Verification items for the finished model (mm, model axes). Face numbers are marked on the shaded views. A direction names the side the tool comes from. Round coordinates to 2 decimals unless told otherwise and drop trailing zeros. Loops run counter-clockwise (first coordinate to the right, second up) from the corner with the lowest first, then second, coordinate; pieces in that order, holes last. Notation, with made-up numbers: M 24,6 L 58,6 A17 cw 58,29 Z; hole C -7,65.5 d7. An arc over 180 degrees is marked long. One line per item, written item: value.
from build123d import *

# Parameters (mm, degrees)
F0_R      = 1.6
F1_DEPTH  = 1.6
F2_W      = 5.5
F2_H      = 10.75
F2_W_2    = 6.8
F2_H_2    = 5.8
F3_DEPTH  = 3.6
F2_W_3    = 8.75
F2_H_3    = 16.2
F4_DEPTH  = 9
F5_DEPTH  = 2
F7_DEPTH  = 2
F6_W      = 8.5
F6_H      = 0.6
F6_H_2    = 9
F8_DEPTH  = 4.25
F6_W_2    = 5.3
F6_H_3    = 6.7
F9_DEPTH  = 3.4
F6_W_3    = 8
F6_H_4    = 7
F10_DEPTH = 4


with BuildPart() as f1:
    # F0 (on Top) → F1 (new body)
    with BuildSketch(Plane.XY):
        with BuildLine():
            Line((15.6, 18.1), (-15.6, 18.1))
            ThreePointArc((-15.6, 18.1), (-17.367767, 17.367767), (-18.1, 15.6))
            Line((-18.1, 15.6), (-18.1, -15.6))
            ThreePointArc((-18.1, -15.6), (-17.367767, -17.367767), (-15.6, -18.1))
            Line((-15.6, -18.1), (15.6, -18.1))
            ThreePointArc((15.6, -18.1), (17.367767, -17.367767), (18.1, -15.6))
            Line((18.1, -15.6), (18.1, 15.6))
            ThreePointArc((18.1, 15.6), (17.367767, 17.367767), (15.6, 18.1))
        make_face()
        with Locations((-15.6, -15.6)):
            Circle(F0_R, mode=Mode.SUBTRACT)
        with Locations((15.6, -15.6)):
            Circle(F0_R, mode=Mode.SUBTRACT)
        with Locations((-15.6, 15.6)):
            Circle(F0_R, mode=Mode.SUBTRACT)
        with Locations((15.6, 15.6)):
            Circle(F0_R, mode=Mode.SUBTRACT)
    extrude(amount=F1_DEPTH)

    # F2 (on face) → F3 (join)
    with BuildSketch(Plane.XY.offset(1.6)):
        with Locations((-15.35, -0.525)):
            Rectangle(F2_W, F2_H)
        with Locations((-6.8, -15.2)):
            Rectangle(F2_W_2, F2_H_2)
        with Locations((6.5, -15.2)):
            Rectangle(F2_W_2, F2_H_2)
    extrude(amount=F3_DEPTH)

    # F2 (on face) → F4 (join)
    with BuildSketch(Plane.XY.offset(1.6)):
        with Locations((13.725, 2.64)):
            Rectangle(F2_W_3, F2_H_3)
    extrude(amount=F4_DEPTH)

    # F2 (on face) → F5 (join)
    with BuildSketch(Plane.XY.offset(1.6)):
        Polygon((-12.6, -5.9), (-18.1, -5.9), (-18.1, -12.6), (-12.6, -12.6), (-12.6, -18.1), (-10.2, -18.1), (-10.2, -12.3), (-3.4, -12.3), (-3.4, -18.1), (3.1, -18.1), (3.1, -12.3), (9.9, -12.3), (9.9, -18.1), (12.6, -18.1), (12.6, -12.6), (18.1, -12.6), (18.1, -5.46), (9.35, -5.46), (9.35, 10.74), (18.1, 10.74), (18.1, 12.6), (12.6, 12.6), (12.6, 18.1), (-12.6, 18.1), (-12.6, 12.6), (-18.1, 12.6), (-18.1, 4.85), (-12.6, 4.85), align=None)
    extrude(amount=F5_DEPTH)

    # F6 (on face) → F7 (join)
    with BuildSketch(Plane(origin=(0, 0, 0), x_dir=(1, 0, 0), z_dir=(0, 0, -1))):
        Polygon((12.8, 12.1), (18.1, 12.1), (18.1, 13.1), (13.1, 13.1), (13.1, 18.1), (4.4, 18.1), (4.4, 9.1), (-4.1, 9.1), (-4.1, 18.1), (-13.1, 18.1), (-13.1, 13.1), (-18.1, 13.1), (-18.1, -13.1), (-13.1, -13.1), (-13.1, -18.1), (-11.3, -18.1), (-11.3, -11.1), (-3.3, -11.1), (-3.3, -18.1), (3.4, -18.1), (3.4, -11.1), (11.4, -11.1), (11.4, -18.1), (13.1, -18.1), (13.1, -13.1), (18.1, -13.1), (18.1, 5.4), (12.8, 5.4), align=None)
    extrude(amount=F7_DEPTH)

    # F6 (on face) → F8 (join)
    with BuildSketch(Plane(origin=(0, 0, 0), x_dir=(1, 0, 0), z_dir=(0, 0, -1))):
        with Locations((0.15, 18.4)):
            Rectangle(F6_W, F6_H)
        with Locations((0.15, 13.6)):
            Rectangle(F6_W, F6_H_2)
    extrude(amount=F8_DEPTH)

    # F6 (on face) → F9 (join)
    with BuildSketch(Plane(origin=(0, 0, 0), x_dir=(1, 0, 0), z_dir=(0, 0, -1))):
        with Locations((15.45, 8.75)):
            Rectangle(F6_W_2, F6_H_3)
    extrude(amount=F9_DEPTH)

    # F6 (on face) → F10 (join)
    with BuildSketch(Plane(origin=(0, 0, 0), x_dir=(1, 0, 0), z_dir=(0, 0, -1))):
        with Locations((7.4, -14.6)):
            Rectangle(F6_W_3, F6_H_4)
        with Locations((-7.3, -14.6)):
            Rectangle(F6_W_3, F6_H_4)
    extrude(amount=F10_DEPTH)


solid = f1.part
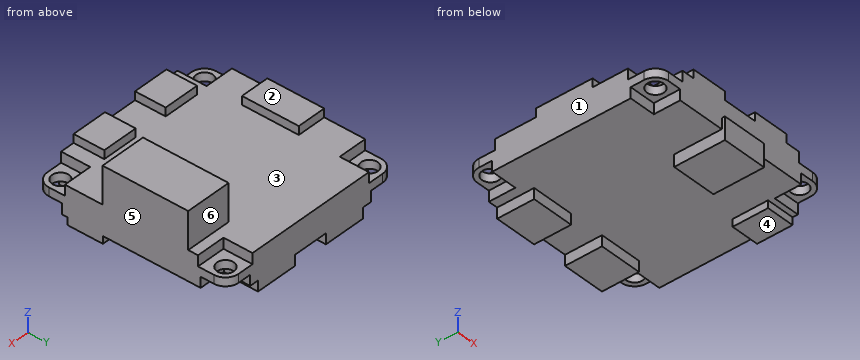
(1) Tool access check on the marked faces 4, 5 and 6. Record the directions out of +Z, -Z, +X, -X, +Y, -Y that give a thin tool (end or side, any length) a straight path to the whole face; none if there is none.
Completed:
face 4: -Z, +X, +Y, -Y
face 5: +Z, -Z, +X, +Y, -Y
face 6: +Z, +X, -X, +Y
(2) Sectioned sample at A-A on y = 0.5. Enter the section's corners in (x, z).
Completed:
outline: M -18.1,-2 L 18.1,-2 L 18.1,10.6 L 9.35,10.6 L 9.35,3.6 L -12.6,3.6 L -12.6,5.2 L -18.1,5.2 Z
(3) Sectioned sample at B-B on x = 1. Enter the section's corners in (y, z).
Completed:
outline: M -18.7,-4.25 L -9.1,-4.25 L -9.1,-2 L 18.1,-2 L 18.1,3.6 L -18.1,3.6 L -18.1,0 L -18.7,0 Z
(4) Sectioned sample at D-D on z = 8.75. Enter the section's corners in (x, y), and give its area (3 significant figures).
Completed:
outline: M 9.35,-5.46 L 18.1,-5.46 L 18.1,10.74 L 9.35,10.74 Z
area: 142 mm^2
(5) Depth check by flat-ended pin: pin 1 Ø1.7 at (x, y) = (5.5, -16) entering from +Z; pin 2 Ø5.5 at (x, y) = (15, 16.5) entering from -Z; pin 3 Ø3.5 at (x, z) = (15, 7) entering from -Y. Enter the tip coordinate at first touch or a pass-through.
Completed:
pin 1: stops at z = 5.2
pin 2: stops at z = -2
pin 3: stops at y = -5.46
(6) Thickness scan on L1, parallel to Y at x = 15.6, z = 1.3; L2, parallel to Y at x = -15, z = 1.5; L3, parallel to Y at x = 15, z = -2.5. Record the ranges inside material, lowest first. Write a range as from..to.
Completed:
L1: y = -18.1..-17.2, -14..14, 17.2..18.1
L2: y = -18.1..-17.08, -14.12..14.12, 17.08..18.1
L3: y = -12.1..-5.4
(7) Sectioned sample at C-C on y = 15. Enter the section's corners in (x, z), and give its area (3 significant figures).
Completed:
outline: M -18.1,0 L -17.08,0 L -17.08,1.6 L -18.1,1.6 Z; M -14.12,0 L -13.1,0 L -13.1,-2 L -11.3,-2 L -11.3,-4 L -3.3,-4 L -3.3,-2 L 3.4,-2 L 3.4,-4 L 11.4,-4 L 11.4,-2 L 13.1,-2 L 13.1,0 L 14.12,0 L 14.12,1.6 L 12.6,1.6 L 12.6,3.6 L -12.6,3.6 L -12.6,1.6 L -14.12,1.6 Z; M 17.08,0 L 18.1,0 L 18.1,1.6 L 17.08,1.6 Z
area: 183 mm^2
(8) Mould release check, pull along X, two halves, no side actions. Record for the marked faces 1, 2 and 3: +X half, -X half, draft (parallel to the pull), parting line (faces both ways), or undercut.
Completed:
face 1: -X half
face 2: draft
face 3: undercut
